```python
from build123d import *

# Parameters (mm, degrees)
SCHIZZO1_W                   = 41
SCHIZZO1_H                   = 28
ESTRUSIONE_ESTRUSIONE1_DEPTH = 1.5
FORO_PER_VITE_M3_1_D         = 3.4
SCHIZZO5_W                   = 6.206252214
SCHIZZO5_H                   = 5.678489494
ESTRUSIONE_ESTRUSIONE2_DEPTH = 1
SCHIZZO6_W                   = 5.958246431
SCHIZZO6_H                   = 6.198352004
ESTRUSIONE_ESTRUSIONE3_DEPTH = 6
SCHIZZO7_W                   = 8.055062412
SCHIZZO7_H                   = 3.777135449
ESTRUSIONE_ESTRUSIONE4_DEPTH = 2


with BuildPart() as part:
    # Schizzo1 → Estrusione-Estrusione1 (new body)
    with BuildSketch(Plane(origin=(0, 0, 0), x_dir=(1, 0, 0), z_dir=(0, 1, 0))):
        Rectangle(SCHIZZO1_W, SCHIZZO1_H)
    extrude(amount=ESTRUSIONE_ESTRUSIONE1_DEPTH)

    # Foro per Vite M3-1 (through all)
    with Locations(Plane(origin=(0, 1.5, 0), x_dir=(1, 0, 0), z_dir=(0, 1, 0))):
        with Locations((17.78, -11.43), (17.78, 11.43), (-17.78, 11.43), (-17.78, -11.43)):
            Hole(FORO_PER_VITE_M3_1_D / 2)

    # Schizzo5 → Estrusione-Estrusione2 (add)
    with BuildSketch(Plane(origin=(0, 1.5, 0), x_dir=(1, 0, 0), z_dir=(0, 1, 0))):
        with Locations((-6.482937483, 1.99695437)):
            Rectangle(SCHIZZO5_W, SCHIZZO5_H)
    extrude(amount=ESTRUSIONE_ESTRUSIONE2_DEPTH)

    # Schizzo6 → Estrusione-Estrusione3 (add)
    with BuildSketch(Plane(origin=(0, 1.5, 0), x_dir=(1, 0, 0), z_dir=(0, 1, 0))):
        with Locations((16.937357628, -4.446973273)):
            Rectangle(SCHIZZO6_W, SCHIZZO6_H)
    extrude(amount=ESTRUSIONE_ESTRUSIONE3_DEPTH)

    # Schizzo7 → Estrusione-Estrusione4 (add)
    with BuildSketch(Plane(origin=(0, 1.5, 0), x_dir=(1, 0, 0), z_dir=(0, 1, 0))):
        with Locations((13.608521834, 5.593352434)):
            Rectangle(SCHIZZO7_W, SCHIZZO7_H)
    extrude(amount=ESTRUSIONE_ESTRUSIONE4_DEPTH)


solid = part.part
```
CAD build for the part. Positions are in the model's coordinates, mm. A direction names the side the tool comes from. Give positions to 0.01 mm unless a question says otherwise; leave off trailing zeros. Write each loop counter-clockwise with the first axis right and the second up, starting at its lowest first coordinate (ties: lowest second). Pieces come first, ordered by that corner, then holes. Notation, with made-up numbers: M -14,22.25 L -3,22.25 A7 cw -3,29.25 Z; hole C 24,85.25 d5. An arc over 180 degrees is marked long. Return JSON: item names as keys, results as strings. Group by question number.
(1) Mould opens along X. For faces 4 (the face through (20.5, 1, 0)), 5 (the face through (17, 7.5, 4)), 6 (the face through (-16.08, 0.74, -11.5)) say: pulls with the +X half, pulls with the -X half, needs draft (parallel to the pull), parting line crosses it, or undercut.
(2) Drill centre lines: L1, parallel to X at y = 0.55, z = 11.43; L2, parallel to Z at x = 17.78, y = 1.05; L3, parallel to Y at x = 19.5, z = -5.5. Where is each one in solid material? Low to high. Write a range as [from, to].
(3) Band-saw the part on A-A (x = -17.78). Give the cut face in (y, z).
(4) Band-saw the part on D-D (x = -7.5). Give the cut face in (y, z).
(5) Flat gauge pins, fed straight in: pin 1 Ø0.6 at (x, y) = (12, 3) entering from -Z; pin 2 Ø1.8 at (x, y) = (16.5, 5.5) entering from +Z; pin 3 Ø14 at (x, z) = (2, 2.5) entering from +Y; pin 4 Ø4 at (y, z) = (2, -1.5) entering from +X. Where does each tip first touch, or does it go through?
(6) 3-axis set-ups, long thin cutter, end or side, ignore diameter. For faces 1 (the face through (-7, 2, 0.842)), 2 (the face through (17, 4, 1.348)), 3 (the face through (19.916, 4, 4)): which of +Z, -Z, +X, -X, +Y, -Y reach the whole face in a straight line?
(7) Band-saw the part on C-C (z = 1.75). Give the cut face in (x, y), and give its area (3 significant figures).
(8) Band-saw the part on B-B (z = 11.43). Give the cut face in (x, y).
Entries:
{
 "1": {"face 4": "pulls with the +X half", "face 5": "needs draft", "face 6": "undercut"},
 "2": {"L1": "x = [-20.5, -19.48], [-16.08, 16.08], [19.48, 20.5]", "L2": "z = [-14, -13.13], [-9.73, 9.73], [13.13, 14]", "L3": "y = [0, 1.5]"},
 "3": {"outline": "M 0,-14 L 1.5,-14 L 1.5,-13.13 L 0,-13.13 Z; M 0,-9.73 L 1.5,-9.73 L 1.5,9.73 L 0,9.73 Z; M 0,13.13 L 1.5,13.13 L 1.5,14 L 0,14 Z"},
 "4": {"outline": "M 0,-14 L 1.5,-14 L 1.5,-4.84 L 2.5,-4.84 L 2.5,0.84 L 1.5,0.84 L 1.5,14 L 0,14 Z"},
 "5": {"pin 1": "stops at z = -7.48", "pin 2": "stops at z = 7.55", "pin 3": "stops at y = 2.5", "pin 4": "stops at x = 20.5"},
 "6": {"face 1": "+Z, +X, -X, +Y", "face 2": "+X, -X, +Y", "face 3": "+Z, -Z, +X, +Y"},
 "7": {"outline": "M -20.5,0 L 20.5,0 L 20.5,1.5 L 19.92,1.5 L 19.92,7.5 L 13.96,7.5 L 13.96,1.5 L -20.5,1.5 Z", "area": "97.2 mm^2"},
 "8": {"outline": "M -20.5,0 L -19.48,0 L -19.48,1.5 L -20.5,1.5 Z; M -16.08,0 L 16.08,0 L 16.08,1.5 L -16.08,1.5 Z; M 19.48,0 L 20.5,0 L 20.5,1.5 L 19.48,1.5 Z"}
}
